Geometry: final body of the model. Coordinates: model frame, mm. A direction names the side the tool comes from. Coordinates: 2 decimals unless noted, no trailing zeros. Order: outer loops, then holes, each group sorted by start corner. A loop starts at its lowest first (then second) coordinate and runs counter-clockwise, first axis right, second up. Notation, with made-up numbers: (-23, 74) -> (26, 74) arc R21 cw to (26, 88) -> close; hole circle Ø5 at (43.25, 77.25). An arc over 180 degrees is marked (long way). Use one line per item in the form item = value.
Autodesk Inventor part; units mm, degrees
ref_plane "YZ Plane" through (0, 0, 0) normal (1, 0, 0) x (0, 1, 0)
ref_plane "XZ Plane" through (0, 0, 0) normal (0, 1, 0) x (-1, 0, 0)
ref_plane "XY Plane" through (0, 0, 0) normal (0, 0, 1) x (1, 0, 0)
sketch "Sketch1" plane through (0, 0, 0) normal (0, 0, 1) x (1, 0, 0)
  arc A0 (4.953, 6.223) -> (0, 6.223) centre (2.4765, 3.2181) ccw
  arc A1 (0, 0.889) -> (4.953, 0.889) centre (2.4765, 3.8939) ccw
  line L0 (0, 6.223) -> (0, 0.889)
  line L1 (4.953, 6.223) -> (4.953, 0.889)
  circle A2 centre (2.4765, 3.556) radius 6.35
  dimension "d26" = 12.7
  dimension "d27" = 5.334
  dimension "d28" = 4.953
  dimension "d29" = 3.8939
  dimension "d30" = 3.8939
  dimension "d31" = 5.334
  dimension "d32" = 2.794
  dimension "d33" = 0.3379
  dimension "d34" = 2.4765
  dimension "d35" = 2.4765
extrude "Extrusion1" add sketch "Sketch1" along normal blind 5.08
sketch "Sketch2" plane through (2.413, 3.4798, 0) normal (0, 0, -1) x (-1, 0, 0)
  circle A0 centre (0, 0) radius 12.7
  circle A1 centre (0, 0) radius 1.0795
  circle A2 centre (0, 0) radius 6.35
  circle A3 centre (0, 9.525) radius 1.0795
  circle A4 centre (0, -9.525) radius 1.0795
  point P0 (2.413, -3.4798)
  dimension "d16" = 25.4
  dimension "d17" = 2.159
  dimension "d18" = 2.159
  dimension "d19" = 2.159
extrude "Extrusion2" add sketch "Sketch2" along normal blind 5.08 contours A0 | A2
properties part number "Zoetrope_Motor_Connector v3"
1) Section D-D, the plane z = -3.75. Output: boundary loops of the cut face in (x, y), and give its area (3 significant figures).
Results found:
outline = circle Ø25.4 at (2.41, 3.48); hole circle Ø2.16 at (2.41, -6.05); hole circle Ø2.16 at (2.41, 3.48); hole circle Ø2.16 at (2.41, 13)
area = 496 mm2
2) Section C-C, the plane y = 9.25. Output: boundary loops of the cut face in (x, z).
Results found:
outline = (-8.9, -5.08) -> (13.73, -5.08) -> (13.73, 0) -> (5.29, 0) -> (5.29, 5.08) -> (-0.33, 5.08) -> (-0.33, 0) -> (-8.9, 0) -> close
3) Access query for faces 5 (the cylindrical face through (-3.447, 14.747, -2.504)), 6 (the cylindrical face through (2.44, 7.11, 2.5)). Directions: +Z, -Z, +X, -X, +Y, -Y. A direction counts if a zero-diameter tool reaches every point of the face in a straight line with its end or side. Return the directions, or none.
Results found:
face_5 = +Z, -Z
face_6 = +Z
4) Section B-B, the plane x = 6. Output: boundary loops of the cut face in (y, z), and give its area (3 significant figures).
Results found:
outline = (-8.7, -5.08) -> (15.66, -5.08) -> (15.66, 0) -> (8.84, 0) -> (8.84, 5.08) -> (-1.73, 5.08) -> (-1.73, 0) -> (-8.7, 0) -> close
area = 177 mm2
5) Contact query for flat-ended pins moving along their axis: P1, Ø1.5, axis at x = 1.5, y = 5, coming from the +Z side; P2, Ø6, axis at y = 12.5, z = -1.5, coming from the +X side; P3, Ø5, axis at x = 9.5, z = -3.5, coming from the -Y side. Output: stop coordinate, or through.
Results found:
P1 = 0
P2 = 13.6
P3 = -8.36
6) Pull-direction query (X, two-part tool) for faces 1 (the flat face through (-3, -2, 0)), 2 (the cylindrical face through (1.1, 9.755, 2.504)), 3 (the cylindrical face through (3.27, 4.137, -2.504)), 4 (the flat face through (4, 4, 0)); classes: released by +X, released by -X, zero draft, split by the parting line, or undercut.
Results found:
face_1 = zero draft
face_2 = split by the parting line
face_3 = undercut
face_4 = undercut
7) Section A-A, the plane y = -5.5. Output: boundary loops of the cut face in (x, z).
Results found:
outline = (-6.57, -5.08) -> (1.48, -5.08) -> (1.48, 0) -> (-6.57, 0) -> close; (3.34, -5.08) -> (11.39, -5.08) -> (11.39, 0) -> (3.34, 0) -> close
8) Material intervals for probe 1 along X at (y, z) = (3.5, -4.25); probe 2 along X at (y, z) = (3.75, 3.75); probe 3 along Y at (x, z) = (2.5, 1), sorted ascending. Write a range as from..to.
Results found:
probe_1 = -10.29..1.33, 3.49..15.11
probe_2 = -3.87..0, 4.95..8.82
probe_3 = -2.79..0, 7.11..9.91
